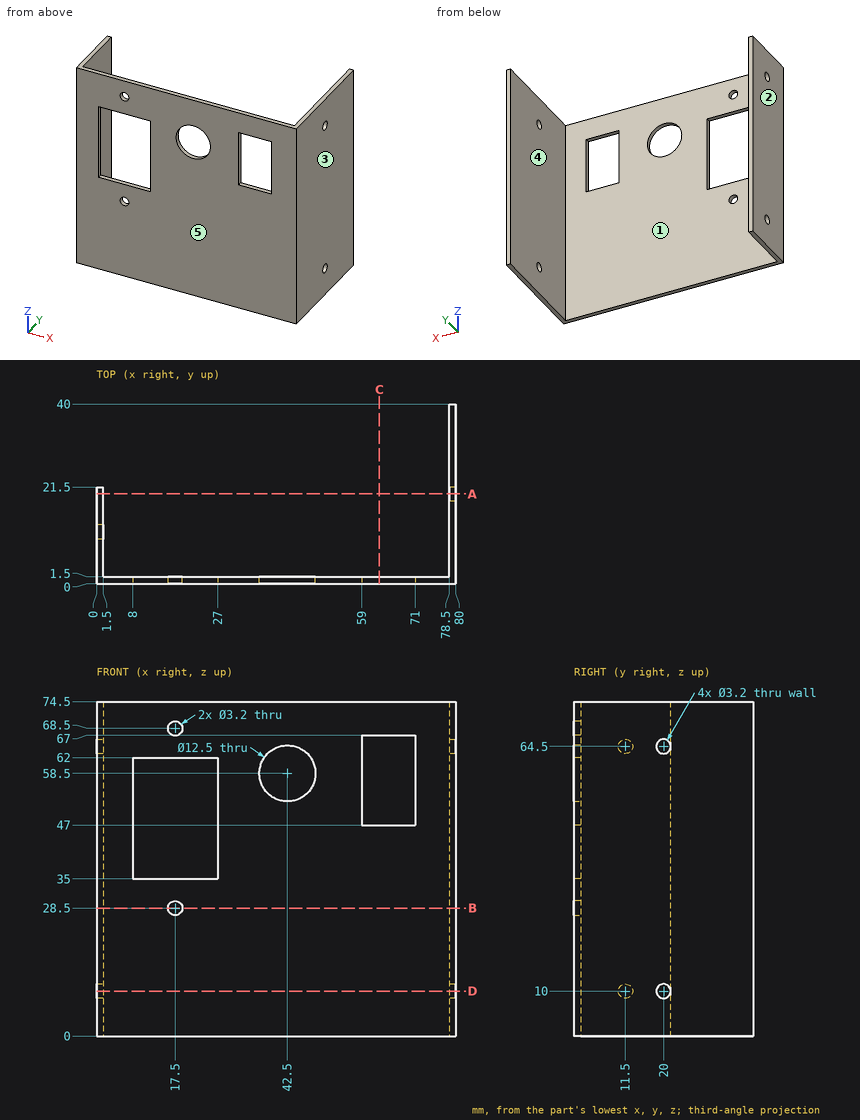
Geometry check sheet. Reference: drawing and pictorial views, mm from the part's lowest x, y, z. A direction names the side the tool comes from. Round coordinates to 2 decimals unless told otherwise and drop trailing zeros. Order: outer loops, then holes, each group sorted by start corner. A loop starts at its lowest first (then second) coordinate and runs counter-clockwise, first axis right, second up. Notation, with made-up numbers: M 42,-34 L 51,-34 A27 ccw 51,-5 Z; hole C 87.5,4.25 d6. An arc over 180 degrees is marked long. Answer as CSV lines item,"result".
1) Sectioned sample at C-C on x = 63. Record the cut outline in (y, z).
Entries:
outline,"M 0,0 L 1.5,0 L 1.5,47 L 0,47 Z; M 0,67 L 1.5,67 L 1.5,74.5 L 0,74.5 Z"
2) Sectioned sample at D-D on z = 10. Record the cut outline in (x, y), and give its area (3 significant figures).
Entries:
outline,"M 0,0 L 80,0 L 80,18.4 L 78.5,18.4 L 78.5,1.5 L 1.5,1.5 L 1.5,9.9 L 0,9.9 Z; M 0,13.1 L 1.5,13.1 L 1.5,21.5 L 0,21.5 Z; M 78.5,21.6 L 80,21.6 L 80,40 L 78.5,40 Z"
area,"198 mm2"
3) Sectioned sample at B-B on z = 28.5. Record the cut outline in (x, y), and give its area (3 significant figures).
Entries:
outline,"M 0,0 L 15.9,0 L 15.9,1.5 L 1.5,1.5 L 1.5,21.5 L 0,21.5 Z; M 19.1,0 L 80,0 L 80,40 L 78.5,40 L 78.5,1.5 L 19.1,1.5 Z"
area,"203 mm2"
4) Sectioned sample at A-A on y = 20. Record the cut outline in (x, z), and give its area (3 significant figures).
Entries:
outline,"M 0,0 L 1.5,0 L 1.5,74.5 L 0,74.5 Z; M 78.5,0 L 80,0 L 80,8.4 L 78.5,8.4 Z; M 78.5,11.6 L 80,11.6 L 80,62.9 L 78.5,62.9 Z; M 78.5,66.1 L 80,66.1 L 80,74.5 L 78.5,74.5 Z"
area,"214 mm2"
5) Tool access check on the marked faces 4 and 5. Record the directions out of +Z, -Z, +X, -X, +Y, -Y that give a thin tool (end or side, any length) a straight path to the whole face; none if there is none.
Entries:
face 4,"+Z, -Z, +Y"
face 5,"+Z, -Z, +X, -X, -Y"
6) Thickness scan on probe 1 along X at (y, z) = (1.15, 58.5); probe 2 along X at (y, z) = (5, 45); probe 3 along Y at (x, z) = (79.55, 64.5). Record the ranges inside material, lowest first. Write a range as [from, to].
Entries:
probe 1,"[0, 8], [27, 36.25], [48.75, 59], [71, 80]"
probe 2,"[0, 1.5], [78.5, 80]"
probe 3,"[0, 18.4], [21.6, 40]"
7) Mould release check, pull along X, two halves, no side actions. Record for the marked faces 1, 2 and 3: +X half, -X half, draft (parallel to the pull), parting line (faces both ways), or undercut.
Entries:
face 1,"undercut"
face 2,"-X half"
face 3,"+X half"
